Source: three-view drawing plus pictorial views. Frame: mm from the lowest corner of the part. Coordinates: 2 decimals unless noted, no trailing zeros. Write each loop counter-clockwise with the first axis right and the second up, starting at its lowest first coordinate (ties: lowest second). Pieces come first, ordered by that corner, then holes. Notation, with made-up numbers: (64.5, -10.75) - (97.5, -10.75) arc R11 ccw to (97.5, -0.75) - close; hole circle Ø5 at (32.25, 62.25). An arc over 180 degrees is marked (long way). Put each result on its own line as item: value.
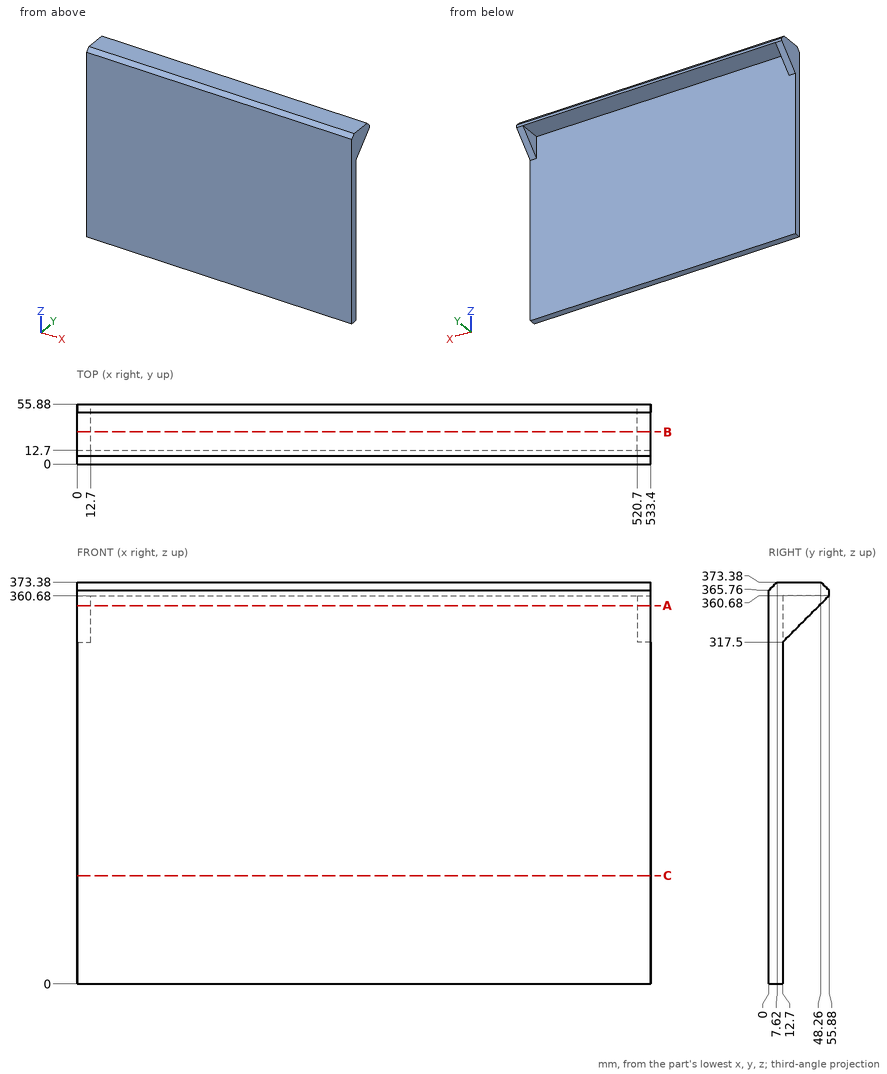
1. Section query C-C (z = 100.5). Return loops of the section in (x, y).
Answer below:
outline: (0, 0) - (533.4, 0) - (533.4, 12.7) - (0, 12.7) - close
2. Section query B-B (y = 30). Return loops of the section in (x, z).
Answer below:
outline: (0, 334.8) - (12.7, 334.8) - (12.7, 360.68) - (520.7, 360.68) - (520.7, 334.8) - (533.4, 334.8) - (533.4, 373.38) - (0, 373.38) - close
3. Section query A-A (z = 351.5). Return loops of the section in (x, y), then the cut area to 3 significant figures.
Answer below:
outline: (0, 0) - (533.4, 0) - (533.4, 46.7) - (520.7, 46.7) - (520.7, 12.7) - (12.7, 12.7) - (12.7, 46.7) - (0, 46.7) - close
area: 7,640 mm²
4. Ray query, probe 1 along Y at (x, z) = (185.5, 208); probe 2 along Z at (x, y) = (176.5, 22). Return the intervals inside material, ascending. Write a range as from..to.
Answer below:
probe 1: y = 0..12.7
probe 2: z = 360.68..373.38
5. Pin query (flat end, axial travel): pin 1 Ø4 at (x, y) = (283, 44.5) entering from -Z; pin 2 Ø6 at (x, z) = (94, 325.5) entering from +Y. Return the tip coordinate at first contact, or that it passes through.
Answer below:
pin 1: stops at z = 360.68
pin 2: stops at y = 12.7
